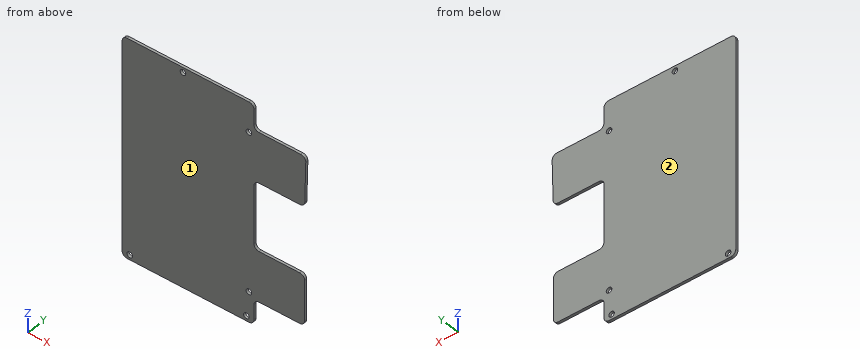
from build123d import *

# Parameters (mm, degrees)
BOSS_EXTRUDE1_DEPTH = 1
SKETCH2_R           = 1.1
CUT_EXTRUDE1_DEPTH  = 4
FILLET1_R           = 2


with BuildPart() as part:
    # Sketch1 → Boss-Extrude1 (new body)
    with BuildSketch(Plane(origin=(0, 0, 0), x_dir=(1, 0, 0), z_dir=(0, 1, 0))):
        Polygon((51.663673174, 77), (51.663673174, 87), (-0.336326826, 87), (-0.336326826, 0), (51.663673174, 0), (51.663673174, 10.002759049), (72.15352325, 10.003966236), (71.663673071, 29.997966506), (51.663673174, 30), (51.663673174, 57), (71.663673174, 57), (71.663673174, 77), align=None)
    extrude(amount=BOSS_EXTRUDE1_DEPTH)

    # Sketch2 → Cut-Extrude1 (cut)
    with BuildSketch(Plane.XZ):
        with Locations((2.663673174, -85)):
            Circle(SKETCH2_R)
        with Locations((48.663673174, -85)):
            Circle(SKETCH2_R)
        with Locations((23.663673174, -2)):
            Circle(SKETCH2_R)
        with Locations((49.663673174, -12.002641219)):
            Circle(SKETCH2_R)
        with Locations((49.663673174, -75)):
            Circle(SKETCH2_R)
    extrude(amount=-CUT_EXTRUDE1_DEPTH, mode=Mode.SUBTRACT)

    # Fillet1
    fillet1_edges = [part.edges().sort_by_distance(p)[0] for p in [
        (-0.336326826, 0.5, -87),
        (51.663673174, 0.5, -87),
        (51.663673174, 0.5, -77),
        (71.663673174, 0.5, -77),
        (71.663673174, 0.5, -57),
        (51.663673174, 0.5, -57),
        (51.663673174, 0.5, -30),
        (71.663673071, 0.5, -29.997966506),
        (72.15352325, 0.5, -10.003966236),
        (51.663673174, 0.5, -10.002759049),
        (51.663673174, 0.5, 0),
        (-0.336326826, 0.5, 0),
    ]]
    fillet(fillet1_edges, radius=FILLET1_R)


solid = part.part
Geometry check sheet. Reference: the model listing, model coordinates, mm. Face numbers are marked on the shaded views. Give positions to 0.01 mm unless a question says otherwise; leave off trailing zeros. Order: outer loops, then holes, each group sorted by start corner. A loop starts at its lowest first (then second) coordinate and runs counter-clockwise, first axis right, second up.
1. Sectioned sample at A-A (y = 0.55). State how many separate pieces and enclosed holes the cut face has, then the cut area to 3 significant figures.
Completed:
separate pieces: 1
enclosed holes: 5
area: 5,310 mm2
2. Draft check along Y on the marked faces 1 and 2. Enter one of: pulls with the +Y half, pulls with the -Y half, needs draft (parallel to the pull), parting line crosses it, or undercut.
Completed:
face 1: pulls with the -Y half
face 2: pulls with the +Y half
3. Sectioned sample at B-B (z = -80). Record the boundary of the cut face in (x, y), then the cut area to 3 significant figures.
Completed:
outline: (-0.34, 0) - (51.66, 0) - (51.66, 1) - (-0.34, 1) - close
area: 52.0 mm2
4. Scan lines: line 1 (X direction, y = 0.3, z = -75); line 2 (Z direction, x = 65, y = 0.65); line 3 (X direction, y = 0.35, z = -85). Record each from-to range of solid material in increasing order.
Completed:
line 1: x = -0.34 to 48.56, 50.76 to 71.66
line 2: z = -77 to -57, -30 to -10
line 3: x = -0.34 to 1.56, 3.76 to 47.56, 49.76 to 51.66
5. Depth check by flat-ended pin: pin 1 (0.5 mm diameter, centred on x = 59, y = 0.5, fed in from -Z); pin 2 (0.5 mm diameter, centred on y = 0.5, z = -5, fed in from +X). Enter the tip coordinate at first touch or a pass-through.
Completed:
pin 1: stops at z = -77
pin 2: stops at x = 51.66
